The drawing under review shows one solid part. Ordinate dimensions are in mm from its lowest x, y, z. Coordinates: 2 decimals unless noted, no trailing zeros. Order: outer loops, then holes, each group sorted by start corner. A loop starts at its lowest first (then second) coordinate and runs counter-clockwise, first axis right, second up. Notation, with made-up numbers: (87, -7) -> (102, -7) arc R28 ccw to (102, 13) -> close; hole circle Ø2 at (34, 86.5). An arc over 180 degrees is marked (long way). Put each result on its own line as item: value.
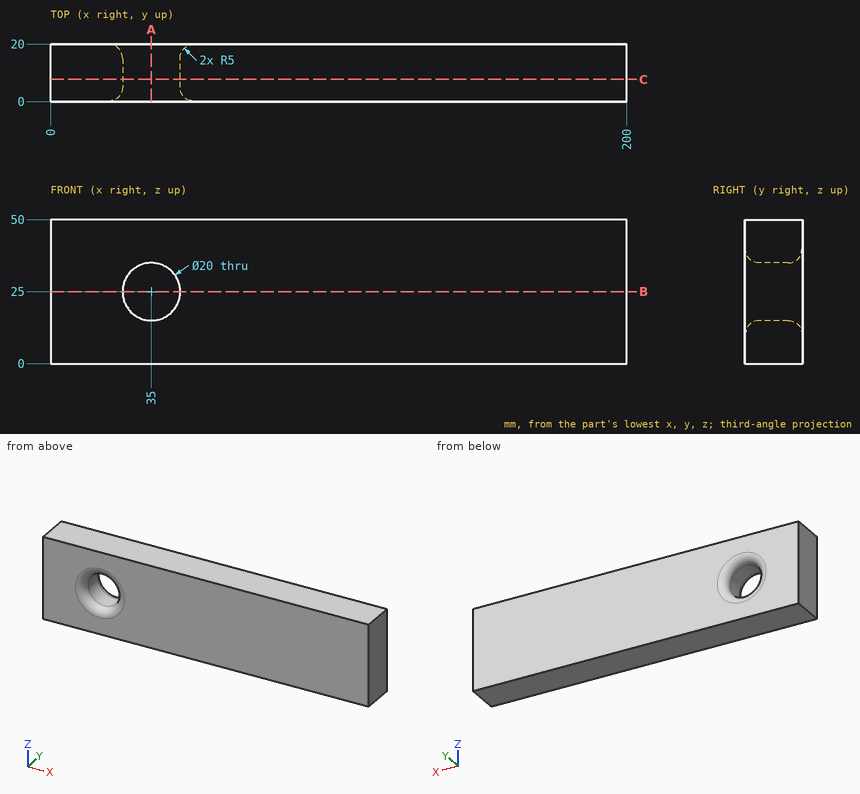
Item 1: Consider section C-C on y = 7.75. Write out the cut boundary in (x, z).
Answers below:
outline: (0, 0) -> (200, 0) -> (200, 50) -> (0, 50) -> close; hole circle Ø20 at (35, 25)
Item 2: For line 1 (Z direction, x = 35, y = 11.5); line 2 (X direction, y = 13.25, z = 24); line 3 (X direction, y = 14, z = 31), list the stretches that pass through material, from the lowest coordinate up. Write a range as from..to.
Answers below:
line 1: 0..15, 35..50
line 2: 0..25.05, 44.95..200
line 3: 0..27, 43..200
Item 3: Consider section A-A on x = 35. Write out the cut boundary in (y, z), and give its area (3 significant figures).
Answers below:
outline: (0, 0) -> (20, 0) -> (20, 10) arc R5 ccw to (15, 15) -> (5, 15) arc R5 ccw to (0, 10) -> close; (0, 40) arc R5 ccw to (5, 35) -> (15, 35) arc R5 ccw to (20, 40) -> (20, 50) -> (0, 50) -> close
area: 579 mm^2
Item 4: Consider section B-B on z = 25. Write out the cut boundary in (x, y), and give its area (3 significant figures).
Answers below:
outline: (0, 0) -> (20, 0) arc R5 ccw to (25, 5) -> (25, 15) arc R5 ccw to (20, 20) -> (0, 20) -> close; (45, 5) arc R5 ccw to (50, 0) -> (200, 0) -> (200, 20) -> (50, 20) arc R5 ccw to (45, 15) -> close
area: 3,580 mm^2
